Design review of the part built by this model. Coordinates are the model's own, in mm. A direction names the side the tool comes from. Give positions to 0.01 mm unless a question says otherwise; leave off trailing zeros. Loops run counter-clockwise (first coordinate to the right, second up) from the corner with the lowest first, then second, coordinate; pieces in that order, holes last. Notation, with made-up numbers: M -26.75,56 L -20.75,56 A10 cw -20.75,71 Z; hole C 37.25,77.5 d9. An arc over 180 degrees is marked long. Use CSV: the item, a comma, the result in double quotes.
from build123d import *

# Parameters (mm, degrees)
CROQUIS1_W               = 49.8
CROQUIS1_H               = 39.8
CROQUIS1_R               = 2.7
SALIENTE_EXTRUIR1_DEPTH  = 6
CORTAR_EXTRUIR1_DEPTH    = 4
REDONDEO1_R              = 3
SALIENTE_EXTRUIR3_DEPTH  = 3
CROQUIS5_R               = 6.35
CORTAR_EXTRUIR2_DEPTH    = 3
SALIENTE_EXTRUIR4_DEPTH  = 10
SALIENTE_EXTRUIR5_DEPTH  = 2
CORTAR_EXTRUIR3_START    = -3
CORTAR_EXTRUIR3_DEPTH    = 3
CORTAR_EXTRUIR4_DEPTH    = 4
CROQUIS10_W              = 4
CROQUIS10_H              = 7
SALIENTE_EXTRUIR6_DEPTH  = 4
CORTAR_EXTRUIR5_START    = -4
CORTAR_EXTRUIR5_DEPTH    = 4
CROQUIS16_W              = 28.958796265
CROQUIS16_H              = 47.870649268
CORTAR_EXTRUIR6_DEPTH    = 2
CROQUIS17_W              = 5
CROQUIS17_H              = 16
CORTAR_EXTRUIR7_DEPTH    = 10
CORTAR_EXTRUIR8_DEPTH    = 2
SALIENTE_EXTRUIR7_DEPTH  = 2
CROQUIS22_R              = 6.5
SALIENTE_EXTRUIR9_DEPTH  = 15
SALIENTE_EXTRUIR10_DEPTH = 1.5
CROQUIS25_W              = 5
CROQUIS25_H              = 15
SALIENTE_EXTRUIR11_DEPTH = 13.5
CROQUIS26_R              = 6
CORTAR_EXTRUIR9_DEPTH    = 5
REDONDEO2_R              = 4


with BuildPart() as part:
    # Croquis1 → Saliente-Extruir1 (new body)
    with BuildSketch(Plane.XY):
        with Locations((-31.963412372, -3.757931034)):
            Rectangle(CROQUIS1_W, CROQUIS1_H)
        with Locations((-52.963412372, 12.342068966)):
            Circle(CROQUIS1_R, mode=Mode.SUBTRACT)
        with Locations((-10.963412372, 12.342068966)):
            Circle(CROQUIS1_R, mode=Mode.SUBTRACT)
        with Locations((-10.963412372, -19.657931034)):
            Circle(CROQUIS1_R, mode=Mode.SUBTRACT)
        with Locations((-52.963412372, -19.657931034)):
            Circle(CROQUIS1_R, mode=Mode.SUBTRACT)
    extrude(amount=SALIENTE_EXTRUIR1_DEPTH)

    # Croquis2 → Cortar-Extruir1 (cut)
    with BuildSketch(Plane.XY.offset(6)):
        with BuildLine():
            Line((-49.963412372, -16.757931034), (-13.963412372, -16.757931034))
            ThreePointArc((-13.963412372, -16.757931034), (-12.54919881, -16.172144597), (-11.963412372, -14.757931034))
            Line((-11.963412372, -14.757931034), (-11.963412372, 7.242068966))
            ThreePointArc((-11.963412372, 7.242068966), (-12.54919881, 8.656282528), (-13.963412372, 9.242068966))
            Line((-13.963412372, 9.242068966), (-49.963412372, 9.242068966))
            ThreePointArc((-49.963412372, 9.242068966), (-51.377625934, 8.656282528), (-51.963412372, 7.242068966))
            Line((-51.963412372, 7.242068966), (-51.963412372, -14.757931034))
            ThreePointArc((-51.963412372, -14.757931034), (-51.377625934, -16.172144597), (-49.963412372, -16.757931034))
        make_face()
    extrude(amount=-CORTAR_EXTRUIR1_DEPTH, mode=Mode.SUBTRACT)

    # Redondeo1
    redondeo1_edges = [part.edges().sort_by_distance(p)[0] for p in [
        (-56.863412372, 16.142068966, 3),
        (-7.063412372, 16.142068966, 3),
        (-7.063412372, -23.657931034, 3),
        (-56.863412372, -23.657931034, 3),
    ]]
    fillet(redondeo1_edges, radius=REDONDEO1_R)

    # Croquis4 → Saliente-Extruir3 (add)
    with BuildSketch(Plane(origin=(0, 0, 0), x_dir=(-1, 0, 0), z_dir=(0, 0, -1))):
        with BuildLine():
            Line((56.863412372, 4.242068966), (61.863412372, 4.242068966))
            Line((61.863412372, 4.242068966), (61.863412372, -0.257931034))
            Line((61.863412372, -0.257931034), (57.863412372, -0.257931034))
            ThreePointArc((57.863412372, -0.257931034), (57.358118834, -0.294597605), (56.863412372, -0.403829068))
            Line((56.863412372, -0.403829068), (56.863412372, 4.242068966))
        make_face()
        with BuildLine():
            Line((61.863412372, -11.757931034), (56.863412372, -11.757931034))
            Line((56.863412372, -11.757931034), (56.863412372, -7.112033001))
            ThreePointArc((56.863412372, -7.112033001), (57.358118834, -7.221264464), (57.863412372, -7.257931034))
            Line((57.863412372, -7.257931034), (61.863412372, -7.257931034))
            Line((61.863412372, -7.257931034), (61.863412372, -11.757931034))
        make_face()
    extrude(amount=-SALIENTE_EXTRUIR3_DEPTH)

    # Croquis5 → Cortar-Extruir2 (cut)
    with BuildSketch(Plane.XY.offset(3)):
        with Locations((-57.863412372, -3.757931034)):
            Circle(CROQUIS5_R)
    extrude(amount=CORTAR_EXTRUIR2_DEPTH, mode=Mode.SUBTRACT)

    # Croquis6 → Saliente-Extruir4 (add)
    with BuildSketch(Plane.XY.offset(3)):
        with BuildLine():
            Line((-61.863412372, 4.242068966), (-51.963412372, 4.242068966))
            Line((-51.963412372, 4.242068966), (-48.963412372, 4.242068966))
            Line((-48.963412372, 4.242068966), (-48.963412372, -11.757931034))
            Line((-48.963412372, -11.757931034), (-51.963412372, -11.757931034))
            Line((-51.963412372, -11.757931034), (-61.863412372, -11.757931034))
            Line((-61.863412372, -11.757931034), (-61.863412372, -8.689715701))
            ThreePointArc((-61.863412372, -8.689715701), (-51.513412372, -3.757931034), (-61.863412372, 1.173853632))
            Line((-61.863412372, 1.173853632), (-61.863412372, 4.242068966))
        make_face()
    extrude(amount=SALIENTE_EXTRUIR4_DEPTH)

    # Croquis7 → Saliente-Extruir5 (add)
    with BuildSketch(Plane.XY.offset(2)):
        Polygon((-51.963412372, -3.757931034), (-51.963412372, 4.242068966), (-48.963412372, 4.242068966), (-48.963412372, -11.757931034), (-51.963412372, -11.757931034), align=None)
    extrude(amount=SALIENTE_EXTRUIR5_DEPTH)

    # Croquis8 → Cortar-Extruir3 (cut)
    with BuildSketch(Plane.XY.offset(3).offset(CORTAR_EXTRUIR3_START)):
        with BuildLine():
            Line((-56.863412372, -0.403829068), (-56.863412372, -7.112033001))
            ThreePointArc((-56.863412372, -7.112033001), (-53.509310406, -3.757931034), (-56.863412372, -0.403829068))
        make_face()
    extrude(amount=CORTAR_EXTRUIR3_DEPTH, mode=Mode.SUBTRACT)

    # Croquis9 → Cortar-Extruir4 (cut)
    with BuildSketch(Plane.XY.offset(6)):
        Polygon((-56.863412372, -11.757931034), (-56.863412372, -27.492217147), (-1.817084798, -27.492217147), (-1.817084798, 22.861833321), (-56.863412372, 22.861833321), (-56.863412372, 4.242068966), (-47.172737702, 4.242068966), (-47.172737702, -11.757931034), align=None)
    extrude(amount=-CORTAR_EXTRUIR4_DEPTH, mode=Mode.SUBTRACT)

    # Croquis10 → Saliente-Extruir6 (add)
    with BuildSketch(Plane.XY.offset(2)):
        with Locations((-9.063412372, 5.842068966)):
            Rectangle(CROQUIS10_W, CROQUIS10_H)
    extrude(amount=SALIENTE_EXTRUIR6_DEPTH)

    # Croquis11 → Cortar-Extruir5 (cut)
    with BuildSketch(Plane(origin=(-7.063412372, 0, 0), x_dir=(0, 0, -1), z_dir=(1, 0, 0)).offset(CORTAR_EXTRUIR5_START)):
        Polygon((-2, 5.842068966), (-2, 7.242068966), (-4, 7.242068966), (-4, 4.442068966), (-2, 4.442068966), align=None)
    extrude(amount=CORTAR_EXTRUIR5_DEPTH, mode=Mode.SUBTRACT)

    # Croquis16 → Cortar-Extruir6 (cut)
    with BuildSketch(Plane.XY.offset(2)):
        with Locations((-49.718694927, -6.990346687)):
            Rectangle(CROQUIS16_W, CROQUIS16_H)
    extrude(amount=CORTAR_EXTRUIR6_DEPTH, mode=Mode.SUBTRACT)


with BuildPart() as cortar_extruir6_kept_piece:
    # of the separate pieces the step leaves, the one the design keeps (cortar_extruir6_pieces_kept)
    add(part.part.solids().sort_by_distance((-53.863412372, 16.142068966, 0))[0])

    # Croquis17 → Cortar-Extruir7 (cut)
    with BuildSketch(Plane.XY.offset(2)):
        with Locations((-59.363412372, -3.757931034)):
            Rectangle(CROQUIS17_W, CROQUIS17_H)
    extrude(amount=-CORTAR_EXTRUIR7_DEPTH, mode=Mode.SUBTRACT)

    # Croquis18 → Cortar-Extruir8 (cut)
    with BuildSketch(Plane.XY.offset(2)):
        with BuildLine():
            Line((-56.863412372, -0.403829068), (-50.513412372, -0.403829068))
            ThreePointArc((-50.513412372, -0.403829068), (-47.159310406, -3.757931034), (-50.513412372, -7.112033001))
            Line((-50.513412372, -7.112033001), (-56.863412372, -7.112033001))
            Line((-56.863412372, -7.112033001), (-56.863412372, -0.403829068))
        make_face()
    extrude(amount=-CORTAR_EXTRUIR8_DEPTH, mode=Mode.SUBTRACT)

    # Croquis20 → Saliente-Extruir7 (add)
    with BuildSketch(Plane.XY.offset(2)):
        with BuildLine():
            Line((-56.863412372, -0.403829068), (-56.863412372, -7.112033001))
            Line((-56.863412372, -7.112033001), (-50.513412372, -7.112033001))
            ThreePointArc((-50.513412372, -7.112033001), (-47.159310406, -3.757931034), (-50.513412372, -0.403829068))
            Line((-50.513412372, -0.403829068), (-56.863412372, -0.403829068))
        make_face()
    extrude(amount=-SALIENTE_EXTRUIR7_DEPTH)

    # Croquis22 → Saliente-Extruir9 (add)
    with BuildSketch(Plane.ZY.offset(56.863412372)):
        with BuildLine():
            Line((2, -3.757931034), (2, 4.742068966))
            Line((2, 4.742068966), (13, 4.742068966))
            ThreePointArc((13, 4.742068966), (15.828427125, 3.57049609), (17, 0.742068966))
            Line((17, 0.742068966), (17, -8.257931034))
            ThreePointArc((17, -8.257931034), (15.828427125, -11.086358159), (13, -12.257931034))
            Line((13, -12.257931034), (2, -12.257931034))
            Line((2, -12.257931034), (2, -3.757931034))
        make_face()
        with Locations(Location((8.55, -3.757931034, 0), (0, 0, 270))):
            Circle(CROQUIS22_R, mode=Mode.SUBTRACT)
    extrude(amount=-SALIENTE_EXTRUIR9_DEPTH)

    # Croquis23 → Saliente-Extruir10 (add)
    with BuildSketch(Plane(origin=(-41.863412372, 0, 0), x_dir=(0, 0, -1), z_dir=(1, 0, 0))):
        with BuildLine():
            Line((-13, -12.257931034), (-2, -12.257931034))
            Line((-2, -12.257931034), (-2, 4.742068966))
            Line((-2, 4.742068966), (-13, 4.742068966))
            ThreePointArc((-13, 4.742068966), (-15.828427125, 3.57049609), (-17, 0.742068966))
            Line((-17, 0.742068966), (-17, -8.257931034))
            ThreePointArc((-17, -8.257931034), (-15.828427125, -11.086358159), (-13, -12.257931034))
        make_face()
    extrude(amount=SALIENTE_EXTRUIR10_DEPTH)

    # Croquis25 → Saliente-Extruir11 (add)
    with BuildSketch(Plane.XY.offset(2)):
        with Locations((-26.563412372, 8.642068966)):
            Rectangle(CROQUIS25_W, CROQUIS25_H)
    extrude(amount=SALIENTE_EXTRUIR11_DEPTH)

    # Croquis26 → Cortar-Extruir9 (cut)
    with BuildSketch(Plane(origin=(-24.063412372, 0, 0), x_dir=(0, 0, -1), z_dir=(1, 0, 0))):
        with Locations((-8.1, 8.642068966)):
            Circle(CROQUIS26_R)
    extrude(amount=-CORTAR_EXTRUIR9_DEPTH, mode=Mode.SUBTRACT)

    # Redondeo2
    redondeo2_edges = [cortar_extruir6_kept_piece.edges().sort_by_distance(p)[0] for p in [
        (-26.563412372, 1.142068966, 15.5),
        (-26.563412372, 16.142068966, 15.5),
    ]]
    fillet(redondeo2_edges, radius=REDONDEO2_R)


solid = cortar_extruir6_kept_piece.part
(1) Clearance check with flat-ended pins moving along their axes: P1, Ø4, axis at y = 5, z = 6.5, coming from the -X side; P2, Ø10, axis at x = -29.5, y = 9, coming from the +Z side; P3, Ø3, axis at x = -40, z = 5, coming from the -Y side; P4, Ø4.5, axis at x = -8.5, z = 4, coming from the +Y side. State where each tip first meets the part, or that it passes through.
A:
P1,"x = -56.86"
P2,"z = 15.5"
P3,"y = -12.26"
P4,"y = 16.09"
(2) The part is to be moulded in two halves that separate along Y. For faces 4 (the flat face through (-40.363, -4, 10)), 5 (the cylindrical face through (-50.388, -18.847, 0.986)), 6 (the cylindrical face through (-56.01, 15.24, 1.01)), say which applies: released by +Y, released by -Y, zero draft, split by the parting line, or undercut.
A:
face 4,"zero draft"
face 5,"undercut"
face 6,"released by +Y"
(3) We need section B-B on x = -36.5. State the section outline as (y, z) points, then the cut area to 3 significant figures.
A:
outline,"M -23.66,0 L 16.14,0 L 16.14,2 L -23.66,2 Z"
area,"79.6 mm²"
(4) Machinability: for faces 1 (the cylindrical face through (-26.528, 2.283, 14.297)), 2 (the flat face through (-49, 4.742, 7)), 3 (the flat face through (-11.063, 5.8, 4.4)), which of the approach directions +Z, -Z, +X, -X, +Y, -Y give a long, thin tool a straight path to every point of the face, cutting with its end or side? Answer none if there is none.
A:
face 1,"+Z, +X, -Y"
face 2,"+Z, -X, +Y"
face 3,"+Z, +Y, -Y"
(5) We need section A-A on z = 7.5. State the section outline as (x, y) points.
A:
outline,"M -56.86,-12.26 L -40.36,-12.26 L -40.36,4.74 L -56.86,4.74 L -56.86,2.66 L -41.86,2.66 L -41.86,-10.17 L -56.86,-10.17 Z; M -29.06,1.14 L -24.06,1.14 L -24.06,2.67 L -29.06,2.67 Z; M -29.06,14.61 L -24.06,14.61 L -24.06,16.14 L -29.06,16.14 Z"
(6) Wall thickness on line 1 along Y through (x, z) = (-10, 2.5); line 2 along Z through (x, y) = (-13, 1); line 3 along X through (y, z) = (-5.5, 6.25): over which ranges is each line inside the solid? List them lowest first. Write a range as [from, to].
A:
line 1,"[2.34, 4.44], [7.24, 9.34]"
line 2,"[0, 2]"
line 3,"[-41.86, -40.36]"
